Can you work these out from the model? Positions are in its coordinate system, mm. A direction names the side the tool comes from. Coordinates: 2 decimals unless noted, no trailing zeros. Write each loop counter-clockwise with the first axis right and the second up, starting at its lowest first coordinate (ties: lowest second). Pieces come first, ordered by that corner, then holes.
```python
from build123d import *

# Parameters (mm, degrees)
SKETCH1_R           = 11
SKETCH1_R_2         = 1.25
BOSS_EXTRUDE1_DEPTH = 5
SKETCH2_R           = 1.35
SKETCH2_R_2         = 1.25
BOSS_EXTRUDE2_DEPTH = 5
FILLET1_R           = 0.5


with BuildPart() as part:
    # Sketch1 → Boss-Extrude1 (new body)
    with BuildSketch(Plane(origin=(0, 0, 0), x_dir=(1, 0, 0), z_dir=(0, 1, 0))):
        with Locations(Location((0, 0, 0), (0, 0, 270))):
            Circle(SKETCH1_R)
        with Locations(Location((0, 7, 0), (0, 0, 270))):
            Circle(SKETCH1_R_2, mode=Mode.SUBTRACT)
        with Locations(Location((7, 0, 0), (0, 0, 270))):
            Circle(SKETCH1_R_2, mode=Mode.SUBTRACT)
        with Locations(Location((0, -7, 0), (0, 0, 270))):
            Circle(SKETCH1_R_2, mode=Mode.SUBTRACT)
        with Locations(Location((-7, 0, 0), (0, 0, 270))):
            Circle(SKETCH1_R_2, mode=Mode.SUBTRACT)
    extrude(amount=BOSS_EXTRUDE1_DEPTH)

    # Sketch2 → Boss-Extrude2 (add)
    with BuildSketch(Plane(origin=(0, 5, 0), x_dir=(1, 0, 0), z_dir=(0, 1, 0))):
        with BuildLine():
            ThreePointArc((-18.75, -16.5), (-18.457106781, -17.207106781), (-17.75, -17.5))
            Line((-17.75, -17.5), (17.75, -17.5))
            ThreePointArc((17.75, -17.5), (18.457106781, -17.207106781), (18.75, -16.5))
            Line((18.75, -16.5), (18.75, 16.5))
            ThreePointArc((18.75, 16.5), (18.457106781, 17.207106781), (17.75, 17.5))
            Line((17.75, 17.5), (-17.75, 17.5))
            ThreePointArc((-17.75, 17.5), (-18.457106781, 17.207106781), (-18.75, 16.5))
            Line((-18.75, 16.5), (-18.75, -16.5))
        make_face()
        with Locations(Location((-13.75, -11.5, 0), (0, 0, 270))):
            Circle(SKETCH2_R, mode=Mode.SUBTRACT)
        with Locations(Location((13.75, -11.5, 0), (0, 0, 270))):
            Circle(SKETCH2_R, mode=Mode.SUBTRACT)
        with Locations(Location((-13.75, 11.5, 0), (0, 0, 270))):
            Circle(SKETCH2_R, mode=Mode.SUBTRACT)
        with Locations(Location((13.75, 11.5, 0), (0, 0, 270))):
            Circle(SKETCH2_R, mode=Mode.SUBTRACT)
        with Locations(Location((0, 7, 0), (0, 0, 270))):
            Circle(SKETCH2_R_2, mode=Mode.SUBTRACT)
        with Locations(Location((0, -7, 0), (0, 0, 270))):
            Circle(SKETCH2_R_2, mode=Mode.SUBTRACT)
        with Locations(Location((-7, 0, 0), (0, 0, 270))):
            Circle(SKETCH2_R_2, mode=Mode.SUBTRACT)
        with Locations(Location((7, 0, 0), (0, 0, 270))):
            Circle(SKETCH2_R_2, mode=Mode.SUBTRACT)
    extrude(amount=BOSS_EXTRUDE2_DEPTH)

    # Fillet1
    fillet1_edges = [part.edges().sort_by_distance(p)[0] for p in [
        (0, 5, -11),
    ]]
    fillet(fillet1_edges, radius=FILLET1_R)


solid = part.part
```
1. If I drill on L1, parallel to X at y = 6.2, z = -11.5; L2, parallel to X at y = 4.75, z = 0; L3, parallel to Y at x = 14, z = 16, over which ranges is the centre line in solid material (lowest first)?
2. If we section it at A-A, the plane z = 0: List the corners of the cut face in (x, y) for me.
3. If we section it at B-B, the plane x = -13.75: List the corners of the cut face in (y, z) for me, plus the area to 3 significant figures.
4. We'd pull the mould along X, two halves only. Please class faces 1 (the face through (-12.411, 7.465, -11.676)), 2 (the face through (0.05, 4.93, 5.75)), 3 (the face through (0, 7, 17.5)), 4 (the face through (18.449, 7.465, 17.215)): released by +X, released by -X, zero draft, split by the parting line, or undercut.
5. If we section it at C-C, the plane y = 6.5: Count the separate pieces of the cut face and the enclosed holes in it, plus the area to 3 significant figures.
6. Which directions (+Z, -Z, +X, -X, +Y, -Y) give clear straight access to the entire face, cutting with the end or side of a thin tool? Please do faces 5 (the face through (0, 5, -12)), 6 (the face through (0, 0, 0)).
7. I'm going to push flat-ended pins straight in: P1, Ø1.5, axis at x = 12.5, z = 5.5, coming from the -Y side; P2, Ø2.5, axis at x = -13.75, z = -11.5, coming from the -Y side; P3, Ø3, axis at y = 2.5, z = 0.5, coming from the -X side. Where does each tip first touch, or does it pass through?
8. If we section it at D-D, the plane y = 2.75: List the corners of the cut face in (x, z) for me, plus the area to 3 significant figures.
Answers:
1. L1: x = -18.75 to -15.1, -12.4 to 12.4, 15.1 to 18.75
1. L2: x = -11.07 to -8.25, -5.75 to 5.75, 8.25 to 11.07
1. L3: y = 5 to 10
2. outline: (-18.75, 5) - (-11.5, 5) arc R0.5 cw to (-11, 4.5) - (-11, 0) - (-8.25, 0) - (-8.25, 10) - (-18.75, 10) - close; (-5.75, 0) - (5.75, 0) - (5.75, 10) - (-5.75, 10) - close; (8.25, 0) - (11, 0) - (11, 4.5) arc R0.5 cw to (11.5, 5) - (18.75, 5) - (18.75, 10) - (8.25, 10) - close
3. outline: (5, -17.5) - (10, -17.5) - (10, -12.85) - (5, -12.85) - close; (5, -10.15) - (10, -10.15) - (10, 10.15) - (5, 10.15) - close; (5, 12.85) - (10, 12.85) - (10, 17.5) - (5, 17.5) - close
3. area: 148 mm2
4. face 1: undercut
4. face 2: undercut
4. face 3: zero draft
4. face 4: released by +X
5. separate pieces: 1
5. enclosed holes: 8
5. area: 1,270 mm2
6. face 5: -Y
6. face 6: +Z, -Z, +X, -X, -Y
7. P1: stops at y = 5
7. P2: passes through
7. P3: stops at x = -11
8. outline: circle Ø22 at (0, 0); hole circle Ø2.5 at (-7, 0); hole circle Ø2.5 at (0, -7); hole circle Ø2.5 at (0, 7); hole circle Ø2.5 at (7, 0)
8. area: 360 mm2
